Check sheet for the modelled part. Datum: model origin and axes. Units: mm. Face numbers are marked on the shaded views. A direction names the side the tool comes from. Give positions to 0.01 mm unless a question says otherwise; leave off trailing zeros. Order: outer loops, then holes, each group sorted by start corner. A loop starts at its lowest first (then second) coordinate and runs counter-clockwise, first axis right, second up.
```python
from build123d import *

# Parameters (mm, degrees)
FILLET1_R     = 1.5875
CHAMFER1_SIZE = 0.635


with BuildPart() as part:
    # Sketch1 → Revolve1 (revolve)
    with BuildSketch(Plane.XY):
        Polygon((0, 0), (1.016, 0), (1.016, 1.27), (1.7145, 1.27), (1.7145, 7.3914), (1.5875, 7.3914), (1.5875, 18.1102), (0, 18.1102), align=None)
    revolve(axis=Axis((0, 0, 0), (0, 1, 0)))

    # Fillet1
    # the kernel refuses this fillet: 1.5875 mm, written as the material it takes off along each edge
    with BuildSketch(Plane(origin=(0, 18.1102, 0), x_dir=(1, 0, 0), z_dir=(0, 0, 1))) as fillet1_piece_1:
        with BuildLine():
            CenterArc((1.5875 - FILLET1_R, -FILLET1_R), FILLET1_R, 0, 90)
            Line((1.5875 - FILLET1_R, 0), (1.5875 - FILLET1_R, FILLET1_R * 0.02))
            Line((1.5875 - FILLET1_R, FILLET1_R * 0.02), (1.5875, FILLET1_R * 0.02))
            Line((1.5875, FILLET1_R * 0.02), (1.5875 + FILLET1_R * 0.02, 0))
            Line((1.5875 + FILLET1_R * 0.02, 0), (1.5875 + FILLET1_R * 0.02, -FILLET1_R))
            Line((1.5875 + FILLET1_R * 0.02, -FILLET1_R), (1.5875, -FILLET1_R))
        make_face()
    revolve(axis=Axis((0, 18.1102, 0), (0, 1, 0)), mode=Mode.SUBTRACT)
    with BuildSketch(Plane(origin=(0, 1.27, 0), x_dir=(1, 0, 0), z_dir=(0, 0, 1))) as fillet1_piece_2:
        with BuildLine():
            CenterArc((0.127, 1.315232014), FILLET1_R, 304.055797743, 55.944202257)
            Line((1.7145, 1.315232014), (1.74625, 1.315232014))
            Line((1.74625, 1.315232014), (1.74625, 0))
            Line((1.74625, 0), (1.7145, -0.03175))
            ThreePointArc((1.7145, -0.03175), (1.36525, -0.03175), (1.03378, -0.02630464))
            Line((1.03378, -0.02630464), (1.016, 0))
        make_face()
    revolve(axis=Axis((0, 1.27, 0), (0, 1, 0)), mode=Mode.SUBTRACT)

    # Chamfer1
    chamfer1_edges = [part.edges().sort_by_distance(p)[0] for p in [
        (-1.016, 0, 0),
    ]]
    chamfer(chamfer1_edges, length=CHAMFER1_SIZE)


solid = part.part
```
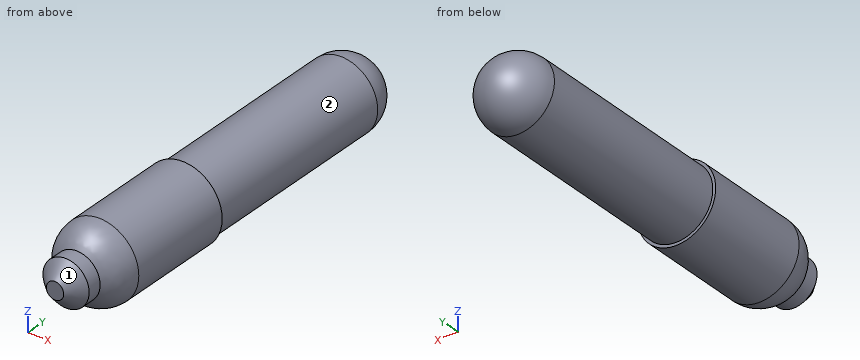
(1) Cross-section at B-B on y = 6.5. Enter the section's corners in (x, z), then the cut area to 3 significant figures.
Response values:
outline: circle Ø3.43 at (0, 0)
area: 9.23 mm2
(2) Gauge pin test, flat end, axial feed: pin 1 Ø1 at (x, z) = (1.5, 0.5) entering from +Y. Record the tip position at first contact, or that the pin passes through.
Response values:
pin 1: stops at y = 17.69
(3) Material ranges on L1, parallel to Z at x = -0.05, y = 13; L2, parallel to X at y = 17.25, z = 1.1; L3, parallel to Z at x = -1.2, y = 7, recorded low to high.
Response values:
L1: z = -1.59 to 1.59
L2: x = -0.88 to 0.88
L3: z = -1.22 to 1.22
(4) Cross-section at A-A on y = 15. Enter the section's corners in (x, z) (1 decimal).
Response values:
outline: circle Ø3.2 at (0, 0)
(5) Set-up check for the marked faces 1 and 2: record each of +Z, -Z, +X, -X, +Y, -Y from which the full face is reachable in a straight line by a thin tool's end or side.
Response values:
face 1: -Y
face 2: +Y
